Build history of the part. All positions in model axes, mm. A direction names the side the tool comes from. Round coordinates to 2 decimals unless told otherwise and drop trailing zeros. Order: outer loops, then holes, each group sorted by start corner. A loop starts at its lowest first (then second) coordinate and runs counter-clockwise, first axis right, second up. Notation, with made-up numbers: (49, 77.25) -> (71, 77.25) arc R19 cw to (71, 82.25) -> close; hole circle Ø5 at (88, -1). An arc over 180 degrees is marked (long way). Write item = value, one per line.
Autodesk Inventor part; units mm, degrees
ref_plane "YZ Plane" through (0, 0, 0) normal (1, 0, 0) x (0, 1, 0)
ref_plane "XZ Plane" through (0, 0, 0) normal (0, 1, 0) x (-1, 0, 0)
ref_plane "XY Plane" through (0, 0, 0) normal (0, 0, 1) x (1, 0, 0)
sketch "Sketch1" plane through (0, 0, 0) normal (0, 0, 1) x (1, 0, 0)
  line L0 (50, -5) -> (50, 23)
  line L1 (50, 23) -> (8, 23)
  line L2 (18, 10) -> (38, 10)
  line L3 (18, 10) -> (18, -5)
  line L4 (38, 10) -> (38, -5)
  line L5 (8, -5) -> (8, 23)
  line L6 (8, -5) -> (18, -5)
  line L7 (38, -5) -> (50, -5)
  dimension "d1" = 28
  dimension "d4" = 15
  dimension "d14" = 20
  dimension "d16" = 12
  dimension "d37" = 42
  dimension "d46" = 28
extrude "Extrusion3" add sketch "Sketch1" along normal blind 10
sketch "Sketch5" plane through (8, -5, 0) normal (0, -1, 0) x (1, 0, 0)
  circle A0 centre (4, 5) radius 2
  line L0 (10, 0) -> (10, 10)
  line L1 (0, 0) -> (10, 0)
  circle A1 centre (36, 5) radius 2
  line L2 (30, 0) -> (30, 10)
  line L3 (30, 0) -> (42, 0)
  dimension "d38" = 4
  dimension "d39" = 6
  dimension "d40" = 5
  dimension "d41" = 4
  dimension "d42" = 6
  dimension "d43" = 5
extrude "Extrusion6" cut sketch "Sketch5" against normal blind 100
properties part number "Espaciador Derecho" material "Aluminum 6061"
Q1. Cut at B-B, the plane x = 44. List the corners of the cut face in (y, z).
Check values:
outline = (-5, 0) -> (23, 0) -> (23, 3) -> (-5, 3) -> close; (-5, 7) -> (23, 7) -> (23, 10) -> (-5, 10) -> close
Q2. Which spindle directions (+Z, -Z, +X, -X, +Y, -Y) get a long thin tool onto all of the face, cutting with end or side? Do faces 4 (the face through (38, 3, 5)), 5 (the face through (43.9, -5, 2.7)). Say none if no direction does.
Check values:
face_4 = +Z, -Z, -Y
face_5 = +Z, -Z, +X, -X, -Y
Q3. Cut at D-D, the plane z = 8.25. List the corners of the cut face in (x, y), and give its area (3 significant figures).
Check values:
outline = (8, -5) -> (18, -5) -> (18, 10) -> (38, 10) -> (38, -5) -> (50, -5) -> (50, 23) -> (8, 23) -> close
area = 876 mm²
Q4. Cut at C-C, the plane z = 5. List the corners of the cut face in (x, y).
Check values:
outline = (8, -5) -> (10, -5) -> (10, 23) -> (8, 23) -> close; (14, -5) -> (18, -5) -> (18, 10) -> (38, 10) -> (38, -5) -> (42, -5) -> (42, 23) -> (14, 23) -> close; (46, -5) -> (50, -5) -> (50, 23) -> (46, 23) -> close
Q5. Probe probe 1 along Z at (x, y) = (44, 8.5); probe 2 along X at (y, z) = (0, 8.5); probe 3 along X at (y, z) = (16.75, 5.25). List the from-to ranges inside material, lowest first.
Check values:
probe_1 = 0 to 3, 7 to 10
probe_2 = 8 to 18, 38 to 50
probe_3 = 8 to 10.02, 13.98 to 42.02, 45.98 to 50
Q6. Flat gauge pins, fed straight in: pin 1 (3 mm diameter, centred on x = 12, z = 5, fed in from +Y); pin 2 (3 mm diameter, centred on x = 31.5, z = 5, fed in from -Y). Where does each tip first touch, or does it go through?
Check values:
pin_1 = through
pin_2 = 10
Q7. Mould opens along X. For faces 1 (the face through (29, 12, 10)), 2 (the face through (28, 10, 5)), 3 (the face through (8, 9, 5)) say: released by +X, released by -X, zero draft, split by the parting line, or undercut.
Check values:
face_1 = zero draft
face_2 = undercut
face_3 = released by -X
Q8. Cut at A-A, the plane y = 2.5. List the corners of the cut face in (x, z).
Check values:
outline = (8, 0) -> (18, 0) -> (18, 10) -> (8, 10) -> close; (38, 0) -> (50, 0) -> (50, 10) -> (38, 10) -> close; hole circle Ø4 at (12, 5); hole circle Ø4 at (44, 5)
